Build history of the part. All positions in model axes, mm. Face numbers are marked on the shaded views. A direction names the side the tool comes from. Round coordinates to 2 decimals unless told otherwise and drop trailing zeros. Write each loop counter-clockwise with the first axis right and the second up, starting at its lowest first coordinate (ties: lowest second). Pieces come first, ordered by that corner, then holes.
Item 1: Mould opens along X. For the marked faces 3 and 4 say: +X half, -X half, draft (parallel to the pull), parting line (faces both ways), or undercut.
Item 2: Drop flat-ended pins along their axis: pin 1 Ø3 at (x, z) = (-4, 34.5) entering from +Y; pin 2 Ø0.5 at (x, y) = (3.5, 1.5) entering from +Z; pin 3 Ø1.1 at (y, z) = (1.5, -33.5) entering from +X. Give the stop position or say it passes through.
Item 3: Band-saw the part on D-D, the plane x = -26.5. Write the cut outline in (y, z), then the cut area to 3 significant figures.
Item 4: Band-saw the part on A-A, the plane z = 0. Write the cut outline in (x, y), then the cut area to 3 significant figures.
Item 5: 3-axis set-ups, long thin cutter, end or side, ignore diameter. For the marked faces 1 and 2: which of +Z, -Z, +X, -X, +Y, -Y reach the whole face in a straight line?
Item 6: Band-saw the part on B-B, the plane x = 0. Write the cut outline in (y, z).
Item 7: Band-saw the part on C-C, the plane y = 1.35. Write the cut outline in (x, z).
Item 8: Wall check: probe 1 along Z at (x, y) = (16, 1.25); probe 2 along X at (y, z) = (1, 2); probe 3 along X at (y, z) = (1.15, 27). Give the ranges that are in metal, low to high.
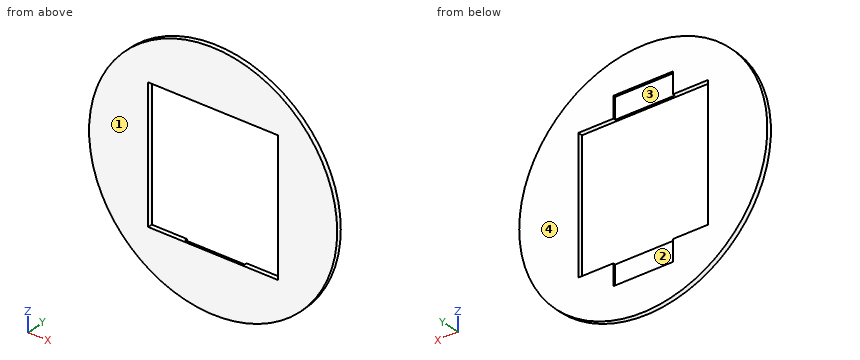
```python
from build123d import *

# Parameters (mm, degrees)
SKETCH1_R           = 54
BOSS_EXTRUDE1_DEPTH = 2
SKETCH2_W           = 56.5
SKETCH2_H           = 58.5
CUT_EXTRUDE1_DEPTH  = 2
SKETCH3_W           = 26
SKETCH3_H           = 9.25
CUT_EXTRUDE2_DEPTH  = 1


with BuildPart() as part:
    # Sketch1 → Boss-Extrude1 (new body)
    with BuildSketch(Plane(origin=(0, 0, 0), x_dir=(1, 0, 0), z_dir=(0, 1, 0))):
        Circle(SKETCH1_R)
    extrude(amount=BOSS_EXTRUDE1_DEPTH)

    # Sketch2 → Cut-Extrude1 (cut)
    with BuildSketch(Plane(origin=(0, 2, 0), x_dir=(1, 0, 0), z_dir=(0, 1, 0))):
        Rectangle(SKETCH2_W, SKETCH2_H)
    extrude(amount=-CUT_EXTRUDE1_DEPTH, mode=Mode.SUBTRACT)

    # Sketch3 → Cut-Extrude2 (cut)
    with BuildSketch(Plane(origin=(0, 2, 0), x_dir=(1, 0, 0), z_dir=(0, 1, 0))):
        with Locations((0, 33.875)):
            Rectangle(SKETCH3_W, SKETCH3_H)
        with Locations((0, -33.875)):
            Rectangle(SKETCH3_W, SKETCH3_H)
    extrude(amount=-CUT_EXTRUDE2_DEPTH, mode=Mode.SUBTRACT)


solid = part.part
```
Results:
1. face 3: undercut
1. face 4: draft
2. pin 1: stops at y = 1
2. pin 2: stops at z = 53.9
2. pin 3: stops at x = 42.78
3. outline: (0, -47.05) - (2, -47.05) - (2, -29.25) - (0, -29.25) - close; (0, 29.25) - (2, 29.25) - (2, 47.05) - (0, 47.05) - close
3. area: 71.2 mm2
4. outline: (-54, 0) - (-28.25, 0) - (-28.25, 2) - (-54, 2) - close; (28.25, 0) - (54, 0) - (54, 2) - (28.25, 2) - close
4. area: 103 mm2
5. face 1: +Z, -Z, +X, -X, -Y
5. face 2: +Y
6. outline: (0, -54) - (2, -54) - (2, -38.5) - (1, -38.5) - (1, -29.25) - (0, -29.25) - close; (0, 29.25) - (1, 29.25) - (1, 38.5) - (2, 38.5) - (2, 54) - (0, 54) - close
7. outline: circle Ø108 at (0, 0); hole (-28.25, -29.25) - (-13, -29.25) - (-13, -38.5) - (13, -38.5) - (13, -29.25) - (28.25, -29.25) - (28.25, 29.25) - (13, 29.25) - (13, 38.5) - (-13, 38.5) - (-13, 29.25) - (-28.25, 29.25) - close
8. probe 1: z = -51.58 to -29.25, 29.25 to 51.58
8. probe 2: x = -53.96 to -28.25, 28.25 to 53.96
8. probe 3: x = -46.77 to -28.25, 28.25 to 46.77
